Autodesk Inventor part; units mm, degrees
ref_plane "YZ Plane" through (0, 0, 0) normal (1, 0, 0) x (0, 1, 0)
ref_plane "XZ Plane" through (0, 0, 0) normal (0, 1, 0) x (-1, 0, 0)
ref_plane "XY Plane" through (0, 0, 0) normal (0, 0, 1) x (1, 0, 0)
sketch "Sketch1" plane through (0, 0, 0) normal (0, 1, 0) x (-1, 0, 0)
  line L0 (0, 0) -> (-20, 0)
  line L1 (-20, 0) -> (-20, 20)
  line L2 (-20, 20) -> (0, 20)
  line L3 (0, 20) -> (0, 0)
  line L4 (-3, 17) -> (-17, 17)
  line L5 (-17, 17) -> (-17, 3)
  line L6 (-17, 3) -> (-3, 3)
  line L7 (-3, 3) -> (-3, 17)
  dimension "d0" = 20
  dimension "d1" = 20
  dimension "d2" = 3
  dimension "d3" = 3
  dimension "d4" = 3
  dimension "d5" = 3
extrude "Extrusion1" add sketch "Sketch1" against normal blind 765
sketch "Sketch2" plane through (20, 0, 20) normal (1, 0, 0) x (0, 0, -1)
  circle A0 centre (10, -8) radius 4
  line L0 (0, 0) -> (20, 0)
  point P0 (10, 0)
  dimension "d8" = 8
  dimension "d9" = 8
extrude "Extrusion2" cut sketch "Sketch2" against normal blind 500
sketch "Sketch3" plane through (20, 0, 0) normal (0, 0, -1) x (-1, 0, 0)
  circle A0 centre (10, -46.5774) radius 1.5
  circle A1 centre (10, -81.5774) radius 1.5
  line L0 (23, -91.5774) -> (-3, -91.5774)
  line L1 (23, -91.5774) -> (23, -36.5774)
  line L2 (-3, -36.5774) -> (23, -36.5774)
  line L3 (-3, -91.5774) -> (-3, -36.5774)
  point P0 (20, 0)
extrude "Extrusion3" cut sketch "Sketch3" against normal blind 10 contours A0 | A1
properties part number "arm"
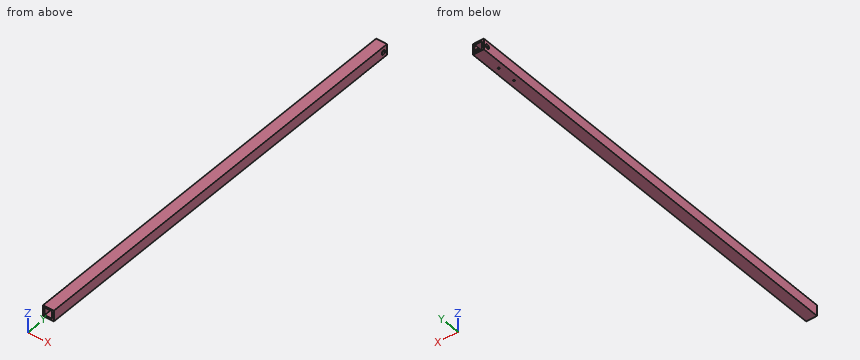
Can you work these out from the model? Positions are in its coordinate system, mm. Coordinates: 2 decimals unless noted, no trailing zeros. Order: outer loops, then holes, each group sorted by start corner. A loop starts at its lowest first (then second) coordinate and runs counter-clockwise, first axis right, second up.
1. If we section it at B-B (z = 10): Please give me the cut outline in (x, y), then the cut area to 3 significant figures.
2. I'm going to push a flat-ended pin straight in: pin 1 (5 mm diameter, centred on y = -8, z = 10, fed in from +X). Where does the tip first touch, or does it pass through?
3. I need wall thicknesses on line 1 (Y direction, x = 10, z = 2.3); line 2 (Z direction, x = 9.25, y = -321.5). Which ranges of each line are inside material? Lowest first, please.
4. If we section it at A-A (y = -489.5): Please give me the cut outline in (x, z).
Entries:
1. outline: (0, -765) - (3, -765) - (3, -12) - (0, -12) - close; (0, -4) - (3, -4) - (3, 0) - (0, 0) - close; (17, -765) - (20, -765) - (20, -12) - (17, -12) - close; (17, -4) - (20, -4) - (20, 0) - (17, 0) - close
1. area: 4,540 mm2
2. pin 1: passes through
3. line 1: y = -765 to -83.08, -80.08 to -48.08, -45.08 to 0
3. line 2: z = 0 to 3, 17 to 20
4. outline: (0, 0) - (20, 0) - (20, 20) - (0, 20) - close; hole (3, 3) - (17, 3) - (17, 17) - (3, 17) - close
